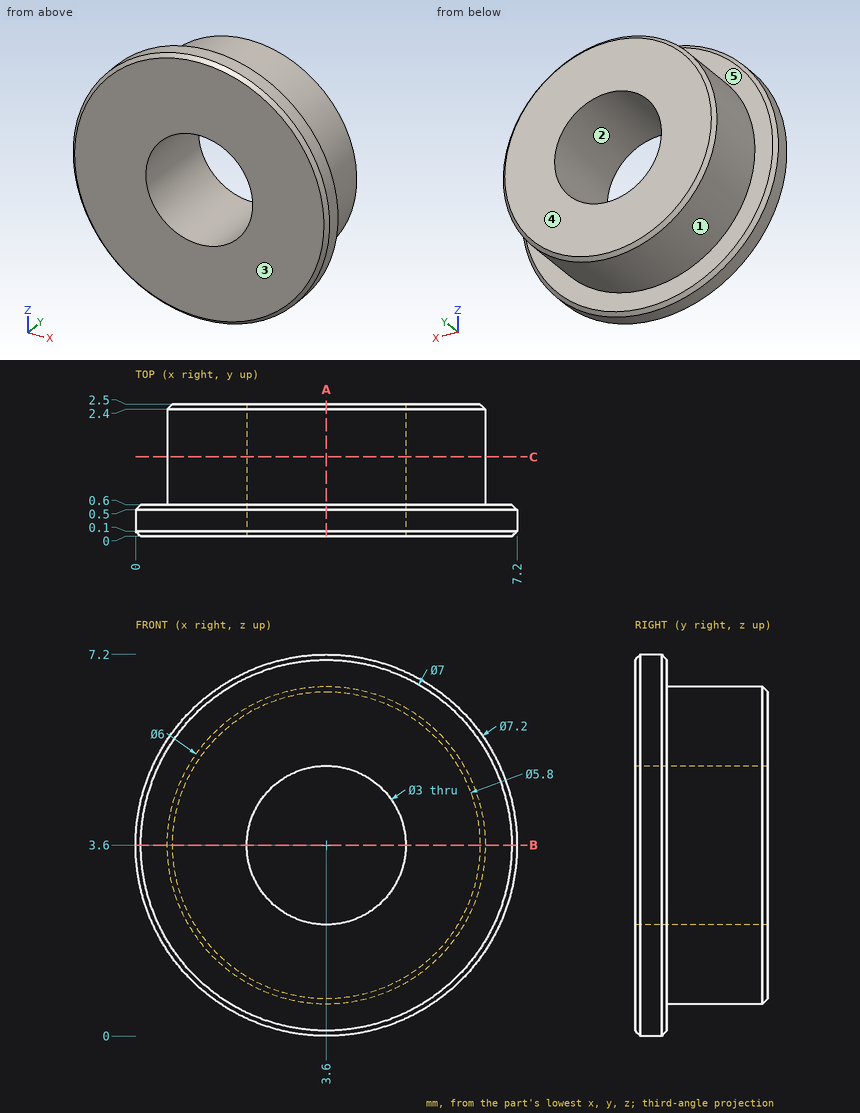
The figure shows three views and two pictorial views of one solid part (mm, origin at its lowest corner). Answer the questions. A direction names the side the tool comes from. Round coordinates to 2 decimals unless told otherwise and drop trailing zeros. Loops run counter-clockwise (first coordinate to the right, second up) from the corner with the lowest first, then second, coordinate; pieces in that order, holes last. Notation, with made-up numbers: (-30.5, 88) - (18.5, 88) arc R9 ccw to (18.5, 94) - close; hole circle Ø6 at (-6, 28.25). An arc over 180 degrees is marked (long way). One line per question, with ' | ' between items. Start each with the question number.
Q1. Section A-A on x = 3.6 is taken. Give the vertices of the cut face in (y, z).
Q2. Find the intervals of material crossed by L1, parallel to X at y = 1.3, z = 3.6; L2, parallel to Z at x = 3.25, y = 1.2; L3, parallel to X at y = 1.9, z = 3, in increasing order.
Q3. Section C-C on y = 1.5 is taken. Give the vertices of the cut face in (x, z), plus the area to 3 significant figures.
Q4. Section B-B on z = 3.6 is taken. Give the vertices of the cut face in (x, y).
Q5. For a pull along X with two mould halves and no side action, classify the marked faces 1, 2 and 3 as +X half, -X half, draft (parallel to the pull), parting line (faces both ways), or undercut.
Q6. For the marked faces 4 and 5, determine the directions among +Z, -Z, +X, -X, +Y, -Y from which every point of the face is accessible in a straight line to the end or side of a thin tool.
Established:
1) outline: (0, 0.1) - (0.1, 0) - (0.5, 0) - (0.6, 0.1) - (0.6, 0.6) - (2.4, 0.6) - (2.5, 0.7) - (2.5, 2.1) - (0, 2.1) - close; (0, 5.1) - (2.5, 5.1) - (2.5, 6.5) - (2.4, 6.6) - (0.6, 6.6) - (0.6, 7.1) - (0.5, 7.2) - (0.1, 7.2) - (0, 7.1) - close
2) L1: 0.6 to 2.1, 5.1 to 6.6 | L2: 0.62 to 2.14, 5.06 to 6.58 | L3: 0.66 to 2.23, 4.97 to 6.54
3) outline: circle Ø6 at (3.6, 3.6); hole circle Ø3 at (3.6, 3.6) | area: 21.2 mm²
4) outline: (0, 0.1) - (0.1, 0) - (2.1, 0) - (2.1, 2.5) - (0.7, 2.5) - (0.6, 2.4) - (0.6, 0.6) - (0.1, 0.6) - (0, 0.5) - close; (5.1, 0) - (7.1, 0) - (7.2, 0.1) - (7.2, 0.5) - (7.1, 0.6) - (6.6, 0.6) - (6.6, 2.4) - (6.5, 2.5) - (5.1, 2.5) - close
5) face 1: parting line | face 2: undercut | face 3: draft
6) face 4: +Z, -Z, +X, -X, +Y | face 5: +Y
